Part model, mm, in its own coordinate system. A direction names the side the tool comes from. Round coordinates to 2 decimals unless told otherwise and drop trailing zeros. Loops run counter-clockwise (first coordinate to the right, second up) from the corner with the lowest first, then second, coordinate; pieces in that order, holes last.
(1) Cut at C-C on x = 14.75. List the corners of the cut face in (y, z), then the cut area to 3 significant figures.
(2) Cut at D-D on z = 6. Count the separate pieces of the cut face and the enclosed holes in it, then the cut area to 3 significant figures.
(3) Cut at A-A on y = 0. List the corners of the cut face in (x, z).
(4) Flat gauge pins, fed straight in: pin 1 (8 mm diameter, centred on y = 0, z = 0.5, fed in from +X); pin 2 (4 mm diameter, centred on x = 16, y = 1.5, fed in from +Z); pin 3 (4 mm diameter, centred on y = 18.5, z = 4, fed in from -X); pin 4 (6 mm diameter, centred on x = 20, z = 15, fed in from +Y). Where does each tip first touch, or does it go through?
(5) Cut at B-B on x = 3. List the corners of the cut face in (y, z) (3 decimals), then the cut area to 3 significant figures.
(6) Probe probe 1 along Y at (x, z) = (19, 0.5); probe 2 along Y at (x, z) = (5.25, -7); probe 3 along Y at (x, z) = (1.5, 8.5). List the from-to ranges inside material, lowest first.
(7) Tool access for faces 3 (the face through (0, 0, 0)), 4 (the face through (2.958, -12.856, 10.593)): list every direction of +Z, -Z, +X, -X, +Y, -Y with a clear straight run to the whole face (end or side of a thin tool).
(8) Mould opens along Y. For faces 1 (the face through (10, 10.3, 0.3)), 2 (the face through (8, 0, -19)) say: +Y half, -Y half, draft (parallel to the pull), parting line (faces both ways), or undercut.
from build123d import *

# Parameters (mm, degrees)
CUT_EXTRUDE_2_DEPTH = 6
CUT_EXTRUDE_3_DEPTH = 26
SKETCH_3_R          = 6.5
CUT_EXTRUDE_4_DEPTH = 15
CHAMFER_1_SIZE      = 1


with BuildPart() as part:
    # Эскиз1 → Повернуть1 (revolve)
    with BuildSketch(Plane.XY):
        Polygon((0, 0), (0, 24), (1, 25), (9, 25), (10, 24), (10, 10), (24, 10), (25, 9), (25, 0), align=None)
    revolve(axis=Axis((0, 0, 0), (1, 0, 0)))

    # Эскиз4 → Вырез-Вытянуть2 (cut)
    with BuildSketch(Plane.ZY):
        with BuildLine():
            ThreePointArc((7.875, 19.467521029), (0, 21), (-7.875, 19.467521029))
            ThreePointArc((-7.875, 19.467521029), (-10.635124054, 12.957396974), (-4.125, 10.19727292))
            ThreePointArc((-4.125, 10.19727292), (0, 11), (4.125, 10.19727292))
            ThreePointArc((4.125, 10.19727292), (10.635124054, 12.957396974), (7.875, 19.467521029))
        make_face()
        with BuildLine():
            ThreePointArc((-10.19727292, 4.125), (-11, 0), (-10.19727292, -4.125))
            ThreePointArc((-10.19727292, -4.125), (-12.957396974, -10.635124054), (-19.467521029, -7.875))
            ThreePointArc((-19.467521029, -7.875), (-21, 0), (-19.467521029, 7.875))
            ThreePointArc((-19.467521029, 7.875), (-12.957396974, 10.635124054), (-10.19727292, 4.125))
        make_face()
        with BuildLine():
            ThreePointArc((-4.125, -10.19727292), (0, -11), (4.125, -10.19727292))
            ThreePointArc((4.125, -10.19727292), (10.635124054, -12.957396974), (7.875, -19.467521029))
            ThreePointArc((7.875, -19.467521029), (0, -21), (-7.875, -19.467521029))
            ThreePointArc((-7.875, -19.467521029), (-10.635124054, -12.957396974), (-4.125, -10.19727292))
        make_face()
    extrude(amount=-CUT_EXTRUDE_2_DEPTH, mode=Mode.SUBTRACT)

    # Эскиз5 → Вырез-Вытянуть3 (cut, through all)
    with BuildSketch(Plane.ZY):
        with BuildLine():
            ThreePointArc((7.125, 17.613471407), (0, 19), (-7.125, 17.613471407))
            ThreePointArc((-7.125, 17.613471407), (-8.781074433, 13.707396974), (-4.875, 12.051322542))
            ThreePointArc((-4.875, 12.051322542), (0, 13), (4.875, 12.051322542))
            ThreePointArc((4.875, 12.051322542), (8.781074433, 13.707396974), (7.125, 17.613471407))
        make_face()
        with BuildLine():
            ThreePointArc((-12.051322542, 4.875), (-13, 0), (-12.051322542, -4.875))
            ThreePointArc((-12.051322542, -4.875), (-13.707396974, -8.781074433), (-17.613471407, -7.125))
            ThreePointArc((-17.613471407, -7.125), (-19, 0), (-17.613471407, 7.125))
            ThreePointArc((-17.613471407, 7.125), (-13.707396974, 8.781074433), (-12.051322542, 4.875))
        make_face()
        with BuildLine():
            ThreePointArc((-4.875, -12.051322542), (0, -13), (4.875, -12.051322542))
            ThreePointArc((4.875, -12.051322542), (8.781074433, -13.707396974), (7.125, -17.613471407))
            ThreePointArc((7.125, -17.613471407), (0, -19), (-7.125, -17.613471407))
            ThreePointArc((-7.125, -17.613471407), (-8.781074433, -13.707396974), (-4.875, -12.051322542))
        make_face()
    extrude(amount=-CUT_EXTRUDE_3_DEPTH, mode=Mode.SUBTRACT)

    # Эскиз3 → Вырез-Вытянуть4 (cut)
    with BuildSketch(Plane(origin=(25, 0, 0), x_dir=(0, 0, -1), z_dir=(1, 0, 0))):
        with Locations((-0.5, 0)):
            Circle(SKETCH_3_R)
    extrude(amount=-CUT_EXTRUDE_4_DEPTH, mode=Mode.SUBTRACT)

    # Фаска1
    chamfer_1_edges = [part.edges().sort_by_distance(p)[0] for p in [
        (25, 0, 7),
    ]]
    chamfer(chamfer_1_edges, length=CHAMFER_1_SIZE)


solid = part.part
Final values:
1. outline: circle Ø20 at (0, 0); hole circle Ø13 at (0, 0.5)
1. area: 181 mm2
2. separate pieces: 3
2. enclosed holes: 0
2. area: 443 mm2
3. outline: (0, -24) - (1, -25) - (9, -25) - (10, -24) - (10, -19) - (6, -19) - (6, -21) - (0, -21) - close; (0, -11) - (6, -11) - (6, -13) - (10, -13) - (10, -10) - (24, -10) - (25, -9) - (25, -7) - (24, -6) - (10, -6) - (10, 7) - (24, 7) - (25, 8) - (25, 9) - (24, 10) - (10, 10) - (10, 24) - (9, 25) - (1, 25) - (0, 24) - close
4. pin 1: stops at x = 10
4. pin 2: stops at z = 10
4. pin 3: stops at x = 6
4. pin 4: passes through
5. outline: circle Ø50 at (0, 0); hole (-19.468, -7.875) arc R5 ccw to (-10.197, -4.125) arc R11 cw to (-10.197, 4.125) arc R5 ccw to (-19.468, 7.875) arc R21 ccw to start; hole (-7.875, -19.468) arc R21 ccw to (7.875, -19.468) arc R5 ccw to (4.125, -10.197) arc R11 cw to (-4.125, -10.197) arc R5 ccw to start; hole (10.197, -4.125) arc R5 ccw to (19.468, -7.875) arc R21 ccw to (19.468, 7.875) arc R5 ccw to (10.197, 4.125) arc R11 cw to start
5. area: 1,360 mm2
6. probe 1: y = -9.99 to -6.5, 6.5 to 9.99
6. probe 2: y = -24 to -19.8, -9.93 to 9.93, 19.8 to 24
6. probe 3: y = -23.51 to -19.16, -10.5 to 10.5, 19.16 to 23.51
7. face 3: +Z, -Z, -X, +Y, -Y
7. face 4: -X
8. face 1: draft
8. face 2: undercut
